Geometry check sheet. Reference: drawing and pictorial views, mm from the part's lowest x, y, z. A direction names the side the tool comes from. Round coordinates to 2 decimals unless told otherwise and drop trailing zeros. Order: outer loops, then holes, each group sorted by start corner. A loop starts at its lowest first (then second) coordinate and runs counter-clockwise, first axis right, second up.
Q1. Depth check by flat-ended pin: P1, Ø1.5, axis at x = 129.5, y = 139.5, coming from the -Z side. Enter the tip coordinate at first touch or a pass-through.
Q2. Cross-section at C-C on z = 164. Record the cut outline in (x, y), then the cut area to 3 significant figures.
Q3. Cross-section at D-D on z = 23. Record the cut outline in (x, y), then the cut area to 3 significant figures.
Q4. Cross-section at B-B on y = 100. Record the cut outline in (x, z).
Q5. Set-up check for the marked faces 1, 2 and 3: record each of +Z, -Z, +X, -X, +Y, -Y from which the full face is reachable in a straight line by a thin tool's end or side.
Q6. Cross-section at A-A on x = 100. Record the cut outline in (y, z).
Q7. Scan lines: probe 1 along Y at (x, z) = (100, 7.25); probe 2 along X at (y, z) = (9, 166.5); probe 3 along Z at (x, y) = (83.5, 135.5). Record each from-to range of solid material in increasing order.
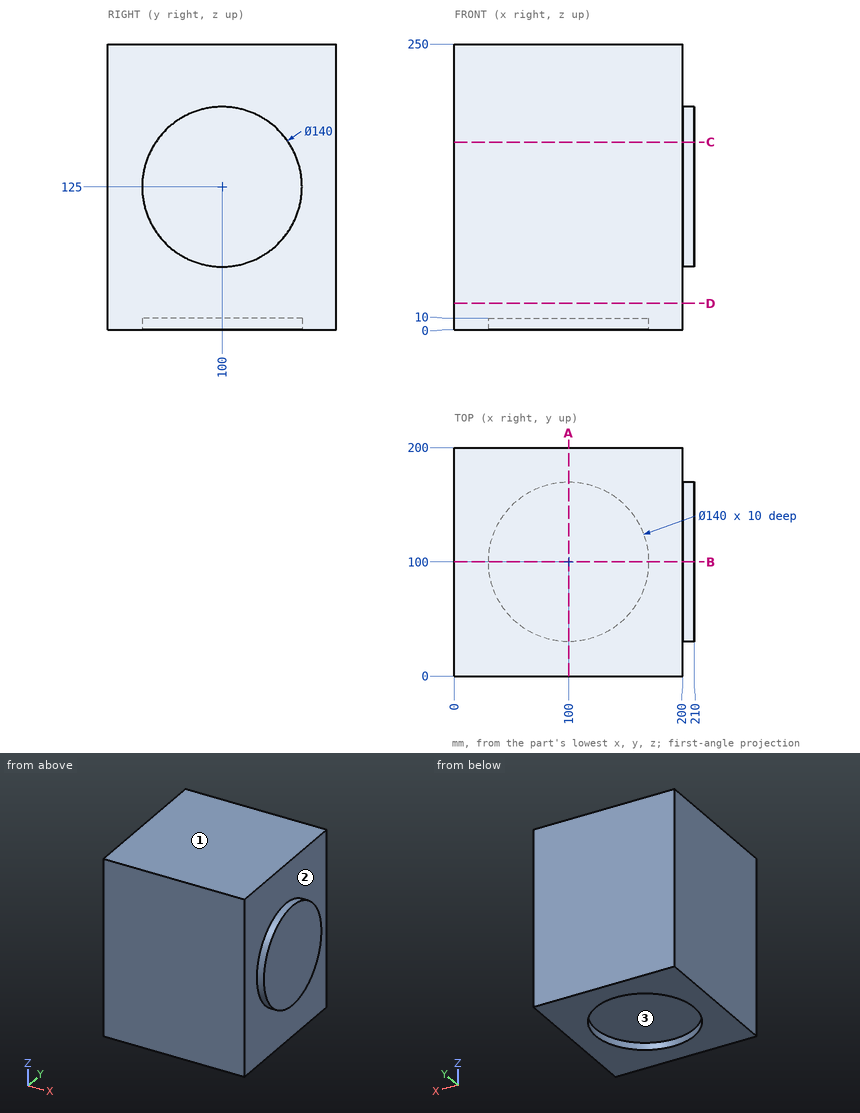
Results found:
1. P1: stops at z = 10
2. outline: (0, 0) - (200, 0) - (200, 41.87) - (210, 41.87) - (210, 158.13) - (200, 158.13) - (200, 200) - (0, 200) - close
2. area: 41,200 mm2
3. outline: (0, 0) - (200, 0) - (200, 200) - (0, 200) - close
3. area: 40,000 mm2
4. outline: (0, 0) - (30, 0) - (30, 10) - (170, 10) - (170, 0) - (200, 0) - (200, 55) - (210, 55) - (210, 195) - (200, 195) - (200, 250) - (0, 250) - close
5. face 1: +Z, +X, -X, +Y, -Y
5. face 2: +X
5. face 3: -Z
6. outline: (0, 0) - (30, 0) - (30, 10) - (170, 10) - (170, 0) - (200, 0) - (200, 250) - (0, 250) - close
7. probe 1: y = 0 to 30, 170 to 200
7. probe 2: x = 0 to 200
7. probe 3: z = 10 to 250
